Geometry: final body of the model. Coordinates: model frame, mm. Face numbers are marked on the shaded views. A direction names the side the tool comes from. Round coordinates to 2 decimals unless told otherwise and drop trailing zeros. Loops run counter-clockwise (first coordinate to the right, second up) from the corner with the lowest first, then second, coordinate; pieces in that order, holes last. Notation, with made-up numbers: (14, -13.75) -> (28, -13.75) arc R21 ccw to (28, 23.25) -> close; hole circle Ø2 at (55.25, 39). An arc over 180 degrees is marked (long way). Answer in a Markdown table with one row per item.
```python
from build123d import *

# Parameters (mm, degrees)
SKETCH2_W           = 30.5
SKETCH2_H           = 56
BOSS_EXTRUDE3_DEPTH = 85
BOSS_EXTRUDE4_DEPTH = 30.5
CUT_EXTRUDE2_DEPTH  = 26
SKETCH5_R           = 2.75
SKETCH5_R_2         = 4.25
SKETCH5_R_3         = 1.75
CUT_EXTRUDE3_DEPTH  = 10
SKETCH7_R           = 11.5
CUT_EXTRUDE5_DEPTH  = 3
SKETCH9_R           = 1.75
CUT_EXTRUDE7_DEPTH  = 77
SKETCH6_R           = 2.5
SKETCH6_R_2         = 1.75
CUT_EXTRUDE8_DEPTH  = 77
BOSS_EXTRUDE5_DEPTH = 10
SKETCH12_W          = 4
SKETCH12_H          = 3
BOSS_EXTRUDE6_DEPTH = 15
FILLET2_R           = 1
SKETCH13_W          = 30.5
SKETCH13_H          = 56
BOSS_EXTRUDE7_DEPTH = 12
CUT_EXTRUDE9_DEPTH  = 22


with BuildPart() as part:
    # Sketch2 → Boss-Extrude3 (new body)
    with BuildSketch(Plane(origin=(0, 0, 0), x_dir=(1, 0, 0), z_dir=(0, 1, 0))):
        with Locations((15.25, -28)):
            Rectangle(SKETCH2_W, SKETCH2_H)
    extrude(amount=BOSS_EXTRUDE3_DEPTH)

    # Sketch4 → Boss-Extrude4 (add)
    with BuildSketch(Plane(origin=(30.5, 0, 0), x_dir=(0, 0, -1), z_dir=(1, 0, 0))):
        with BuildLine():
            Line((-56, 85), (0, 85))
            ThreePointArc((0, 85), (-28, 113), (-56, 85))
        make_face()
    extrude(amount=-BOSS_EXTRUDE4_DEPTH)

    # Sketch3 → Cut-Extrude2 (cut)
    with BuildSketch(Plane.ZY):
        with BuildLine():
            Line((5, 10), (5, 80))
            Line((5, 80), (5, 85))
            ThreePointArc((5, 85), (28, 108), (51, 85))
            Line((51, 85), (51, 80))
            Line((51, 80), (51, 10))
            Line((51, 10), (51, 7))
            Line((51, 7), (5, 7))
            Line((5, 7), (5, 10))
        make_face()
    extrude(amount=-CUT_EXTRUDE2_DEPTH, mode=Mode.SUBTRACT)

    # Sketch5 → Cut-Extrude3 (cut)
    with BuildSketch(Plane.ZY.offset(-26)):
        with Locations((28, 20)):
            Circle(SKETCH5_R)
        with Locations((28, 79.06)):
            Circle(SKETCH5_R_2)
        with Locations((28, 52)):
            Circle(SKETCH5_R_3)
    extrude(amount=-CUT_EXTRUDE3_DEPTH, mode=Mode.SUBTRACT)

    # Sketch7 → Cut-Extrude5 (cut)
    with BuildSketch(Plane(origin=(30.5, 0, 0), x_dir=(0, 0, -1), z_dir=(1, 0, 0))):
        with Locations((-28, 20)):
            Circle(SKETCH7_R)
    extrude(amount=-CUT_EXTRUDE5_DEPTH, mode=Mode.SUBTRACT)

    # Sketch9 → Cut-Extrude7 (cut)
    with BuildSketch(Plane.ZY):
        with Locations((5, 3.5)):
            Circle(SKETCH9_R)
        with Locations((51, 3.5)):
            Circle(SKETCH9_R)
    extrude(amount=-CUT_EXTRUDE7_DEPTH, mode=Mode.SUBTRACT)

    # Sketch6 → Cut-Extrude8 (cut)
    with BuildSketch(Plane(origin=(30.5, 0, 0), x_dir=(0, 0, -1), z_dir=(1, 0, 0))):
        with Locations((-49.92, 20)):
            Circle(SKETCH6_R)
        with Locations((-6.08, 20)):
            Circle(SKETCH6_R)
        with Locations((-28, 41.92)):
            Circle(SKETCH6_R_2)
    extrude(amount=-CUT_EXTRUDE8_DEPTH, mode=Mode.SUBTRACT)

    # Sketch11 → Boss-Extrude5 (add)
    with BuildSketch(Plane.XY.offset(56)):
        Polygon((15.25, 2.5), (17.25, 2.5), (17.25, 0), (15.25, 0), (13.25, 0), (13.25, 2.5), align=None)
    extrude(amount=BOSS_EXTRUDE5_DEPTH)

    # Sketch12 → Boss-Extrude6 (add)
    with BuildSketch(Plane.XZ):
        with Locations((15.25, 64.5)):
            Rectangle(SKETCH12_W, SKETCH12_H)
    extrude(amount=BOSS_EXTRUDE6_DEPTH)

    # Fillet2
    fillet2_edges = [part.edges().sort_by_distance(p)[0] for p in [
        (17.25, 1.25, 56),
        (15.25, 2.5, 56),
        (17.25, 2.5, 61),
        (13.25, 1.25, 56),
        (13.25, 2.5, 61),
        (15.25, 2.5, 66),
        (15.25, 0, 63),
        (13.25, -15, 64.5),
        (17.25, -15, 64.5),
    ]]
    fillet(fillet2_edges, radius=FILLET2_R)

    # Sketch13 → Boss-Extrude7 (add)
    with BuildSketch(Plane.XZ):
        with Locations((15.25, 28)):
            Rectangle(SKETCH13_W, SKETCH13_H)
        with BuildLine():
            Line((8.34810103, 28.004718314), (12.411901595, 23.940917749))
            Line((12.411901595, 23.940917749), (16.65189897, 28.180915124))
            Line((16.65189897, 28.180915124), (12.592816719, 32.239997375))
            ThreePointArc((12.592816719, 32.239997375), (9.593303861, 31.001467248), (8.34810103, 28.004718314))
        make_face(mode=Mode.SUBTRACT)
    extrude(amount=BOSS_EXTRUDE7_DEPTH)

    # Sketch15 → Cut-Extrude9 (cut)
    with BuildSketch(Plane.XZ.offset(12)):
        with BuildLine():
            Line((8.34810103, 28.004718314), (12.411901595, 23.940917749))
            Line((12.411901595, 23.940917749), (16.65189897, 28.180915124))
            Line((16.65189897, 28.180915124), (12.592816719, 32.239997375))
            ThreePointArc((12.592816719, 32.239997375), (9.593303861, 31.001467248), (8.34810103, 28.004718314))
        make_face()
    extrude(amount=-CUT_EXTRUDE9_DEPTH, mode=Mode.SUBTRACT)


solid = part.part
```
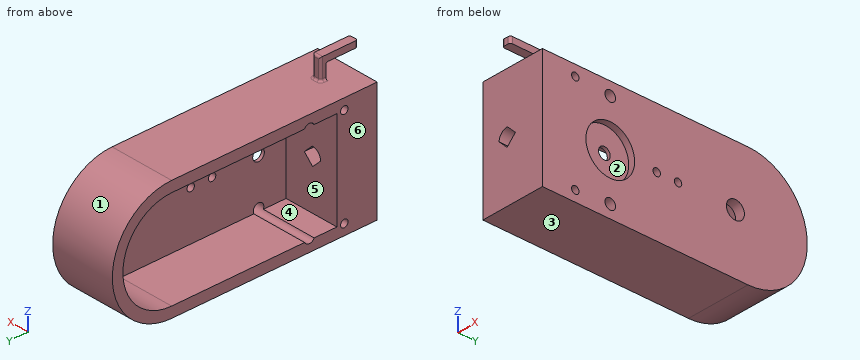
Item 1: Set-up query: the marked faces 5 and 6. Return all of +Z, -Z, +X, -X, +Y, -Y with unobstructed straight access to the full face (end or side cutting, diameter ignored); none if empty.
Ans:
| item | result |
|---|---|
| face 5 | -X |
| face 6 | +Z, -Z, -X, +Y, -Y |
Item 2: Section query C-C, the plane y = 20. Output: boundary loops of the cut face in (x, z), and give its area (3 significant figures).
Ans:
| item | result |
|---|---|
| outline | (0, 0) -> (30.5, 0) -> (30.5, 3.58) -> (0, 3.58) -> close; (0, 52.42) -> (30.5, 52.42) -> (30.5, 56) -> (0, 56) -> close; (26, 8.58) -> (30.5, 8.58) -> (30.5, 16.5) -> (27.5, 16.5) -> (27.5, 25.25) -> (26, 25.25) -> close; (26, 30.75) -> (27.5, 30.75) -> (27.5, 39.5) -> (30.5, 39.5) -> (30.5, 47.42) -> (26, 47.42) -> close |
| area | 316 mm2 |
Item 3: Section query B-B, the plane x = 7. Output: boundary loops of the cut face in (y, z).
Ans:
| item | result |
|---|---|
| outline | (-12, 0) -> (85, 0) arc R28 ccw to (85, 56) -> (-12, 56) -> close; hole circle Ø3.5 at (3.5, 5); hole circle Ø3.5 at (3.5, 51); hole (7, 5) -> (17.75, 5) arc R2.5 ccw to (22.25, 5) -> (85, 5) arc R23 ccw to (85, 51) -> (22.25, 51) arc R2.5 ccw to (17.75, 51) -> (7, 51) -> close |
Item 4: First-contact query: P1, Ø13, axis at x = 11, z = 28.5, coming from the +Y side; P2, Ø7, axis at y = -4, z = 60, coming from the -X side; P3, Ø10, axis at x = 10.5, y = 90.5, coming from the -Z side. Flat tips, straight axial feed; report the tip coordinate or a pass-through.
Ans:
| item | result |
|---|---|
| P1 | y = 113 |
| P2 | x = 13.25 |
| P3 | z = 0 |
Item 5: Ray query, L1, parallel to Y at x = 27, z = 28; L2, parallel to Y at x = 29.45, z = 28; L3, parallel to Z at x = 16, y = 20. Return the intervals inside material, ascending.
Ans:
| item | result |
|---|---|
| L1 | -12 to 17.25, 22.75 to 40.17, 43.67 to 50.25, 53.75 to 74.81, 83.31 to 113 |
| L2 | -12 to 8.5, 31.5 to 40.17, 43.67 to 50.25, 53.75 to 74.81, 83.31 to 113 |
| L3 | 0 to 3.58, 52.42 to 56 |
Item 6: Section query A-A, the plane y = 79.06. Output: boundary loops of the cut face in (x, z), and give its area (3 significant figures).
Ans:
| item | result |
|---|---|
| outline | (0, 0) -> (30.5, 0) -> (30.5, 23.75) -> (26, 23.75) -> (26, 5) -> (0, 5) -> close; (0, 51) -> (26, 51) -> (26, 32.25) -> (30.5, 32.25) -> (30.5, 56) -> (0, 56) -> close |
| area | 474 mm2 |
Item 7: Section query D-D, the plane y = 56.5. Output: boundary loops of the cut face in (x, z).
Ans:
| item | result |
|---|---|
| outline | (0, 0) -> (30.5, 0) -> (30.5, 56) -> (0, 56) -> (0, 51) -> (26, 51) -> (26, 5) -> (0, 5) -> close |
Item 8: Mould query, pull axis Y, two halves, no side actions, for the marked faces 1, 2, 3 and 4. Classes: released by +Y, released by -Y, zero draft, split by the parting line, or undercut.
Ans:
| item | result |
|---|---|
| face 1 | released by +Y |
| face 2 | undercut |
| face 3 | zero draft |
| face 4 | undercut |
